The figure shows three views and two pictorial views of one solid part (mm, origin at its lowest corner). Answer the questions. Coordinates: 2 decimals unless noted, no trailing zeros. Write each loop counter-clockwise with the first axis right and the second up, starting at its lowest first coordinate (ties: lowest second). Pieces come first, ordered by that corner, then holes. Notation, with made-up numbers: M 37.25,33.25 L 59.25,33.25 A30 cw 59.25,55.25 Z; hole C 84,27 d4. An arc over 180 degrees is marked long. Write item = value, one per line. Start each with the question number.
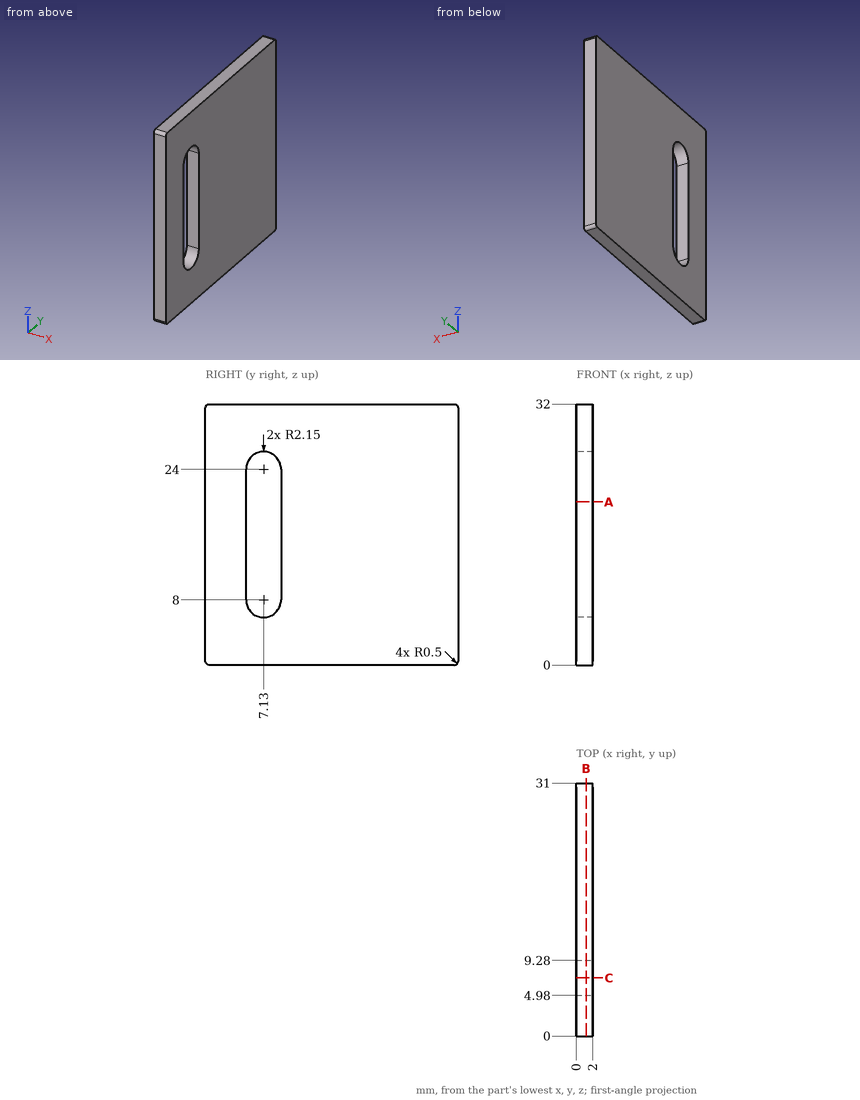
1. Straight lines are drawn through the part: L1, parallel to Y at x = 0.5, z = 12.5; L2, parallel to Y at x = 0.15, z = 25; L3, parallel to Z at x = 0.2, y = 8. For each, find the intervals that lie inside material, in ascending order. Write a range as [from, to].
2. The part is cut by section B-B, the plane x = 1.2. Write down the section's boundary in (y, z), and give its area (3 significant figures).
3. The part is cut by section C-C, the plane y = 7.13. Write down the section's boundary in (x, z).
4. The part is cut by section A-A, the plane z = 20. Write down the section's boundary in (x, y).
Solution:
q1.L1 = [0, 4.98], [9.28, 31]
q1.L2 = [0, 5.23], [9.03, 31]
q1.L3 = [0, 6.03], [25.97, 32]
q2.outline = M 0,0.5 A0.5 ccw 0.5,0 L 30.5,0 A0.5 ccw 31,0.5 L 31,31.5 A0.5 ccw 30.5,32 L 0.5,32 A0.5 ccw 0,31.5 Z; hole M 4.98,8 A2.15 ccw 9.28,8 L 9.28,24 A2.15 ccw 4.98,24 Z
q2.area = 908 mm^2
q3.outline = M 0,0 L 2,0 L 2,5.85 L 0,5.85 Z; M 0,26.15 L 2,26.15 L 2,32 L 0,32 Z
q4.outline = M 0,0 L 2,0 L 2,4.98 L 0,4.98 Z; M 0,9.28 L 2,9.28 L 2,31 L 0,31 Z
